Autodesk Inventor part; units mm, degrees
ref_plane "FDT_FRONT_XY" through (33, 0, 0) normal (1, 0, 0) x (0, 0, -1)
ref_plane "FDT_FRONT_YZ" through (33, 0, 0) normal (0, 0, -1) x (0, 1, 0)
ref_plane "FDT_FRONT_ZX" through (33, 0, 0) normal (0, 1, 0) x (1, 0, 0)
sketch "Sketch_22" plane through (0, 0, 0) normal (0, 0, 1) x (1, 0, 0)
  line L0 (33, 0) -> (0, 0)
  line L1 (0, 0) -> (0, 20.8)
  line L2 (0, 20.8) -> (0.6, 21.4)
  line L3 (0.6, 21.4) -> (3, 21.4)
  line L4 (3, 21.4) -> (3.6351, 22.5)
  line L5 (3.6351, 22.5) -> (27.3649, 22.5)
  line L6 (27.3649, 22.5) -> (27.8268, 21.7)
  arc A0 (27.8268, 21.7) -> (28.3464, 21.4) centre (28.3464, 22) ccw
  line L7 (28.3464, 21.4) -> (29.4, 21.4)
  arc A1 (29.4, 21.4) -> (30, 22) centre (29.4, 22) ccw
  line L8 (30, 22) -> (30, 22.5)
  line L9 (30, 22.5) -> (33, 22.5)
  line L10 (33, 22.5) -> (33, 0)
  line L11 (33, 0) -> (0, 0)
revolve "Revolution1" add sketch "Sketch_22" angle 360 about axis through (33, 0, 0) along (1, 0, 0)
thread "Thread1"
sketch "Sketch_2" plane through (33, 0, 0) normal (1, 0, 0) x (0, 0, -1)
  arc A0 (-12.7904, 32.5792) -> (12.7904, 32.5792) centre (0, 0) ccw
  arc A1 (12.6, 32.8585) -> (12.7904, 32.5792) centre (12.9, 32.8585) ccw
  line L0 (12.6, 32.8585) -> (12.6, 34.8)
  arc A2 (12.6, 34.8) -> (12.4, 35) centre (12.4, 34.8) ccw
  line L1 (12.4, 35) -> (-12.4, 35)
  arc A3 (-12.4, 35) -> (-12.6, 34.8) centre (-12.4, 34.8) ccw
  line L2 (-12.6, 34.8) -> (-12.6, 32.8585)
  arc A4 (-12.7904, 32.5792) -> (-12.6, 32.8585) centre (-12.9, 32.8585) ccw
extrude "Extrusion1" add sketch "Sketch_2" along normal blind 28
sketch "Sketch_3" plane through (0, 0, 0) normal (0, 0, 1) x (1, 0, 0)
  line L0 (599.2, 0) -> (61, 0)
  line L1 (61, 0) -> (61, 32.7)
  line L2 (61, 32.7) -> (599.2, 32.7)
  line L3 (599.2, 32.7) -> (599.2, 0)
  line L4 (599.2, 0) -> (61, 0)
revolve "Revolution2" add sketch "Sketch_3" angle 360 about axis through (599.2, 0, 0) along (1, 0, 0)
sketch "Sketch_16" plane through (599.2, 0, 0) normal (1, 0, 0) x (0, 0, -1)
  arc A0 (-12.7904, 32.5792) -> (12.7904, 32.5792) centre (0, 0) ccw
  arc A1 (12.6, 32.8585) -> (12.7904, 32.5792) centre (12.9, 32.8585) ccw
  line L0 (12.6, 32.8585) -> (12.6, 34.8)
  arc A2 (12.6, 34.8) -> (12.4, 35) centre (12.4, 34.8) ccw
  line L1 (12.4, 35) -> (-12.4, 35)
  arc A3 (-12.4, 35) -> (-12.6, 34.8) centre (-12.4, 34.8) ccw
  line L2 (-12.6, 34.8) -> (-12.6, 32.8585)
  arc A4 (-12.7904, 32.5792) -> (-12.6, 32.8585) centre (-12.9, 32.8585) ccw
extrude "Extrusion2" add sketch "Sketch_16" along normal blind 28
sketch "Sketch_5" plane through (0, 0, 0) normal (0, 0, 1) x (1, 0, 0)
  line L0 (660.2, 0) -> (627.2, 0)
  line L1 (627.2, 0) -> (627.2, 22.5)
  line L2 (627.2, 22.5) -> (630.2, 22.5)
  line L3 (630.2, 22.5) -> (630.2, 22)
  arc A0 (630.2, 22) -> (630.8, 21.4) centre (630.8, 22) ccw
  line L4 (630.8, 21.4) -> (631.8536, 21.4)
  arc A1 (631.8536, 21.4) -> (632.3732, 21.7) centre (631.8536, 22) ccw
  line L5 (632.3732, 21.7) -> (632.8351, 22.5)
  line L6 (632.8351, 22.5) -> (656.5649, 22.5)
  line L7 (656.5649, 22.5) -> (657.2, 21.4)
  line L8 (657.2, 21.4) -> (659.6, 21.4)
  line L9 (659.6, 21.4) -> (660.2, 20.8)
  line L10 (660.2, 20.8) -> (660.2, 0)
  line L11 (660.2, 0) -> (627.2, 0)
revolve "Revolution3" add sketch "Sketch_5" angle 360 about axis through (660.2, 0, 0) along (1, 0, 0)
thread "Thread2"
sketch "Sketch_6" plane through (0, 0, 0) normal (0, 1, 0) x (-1, 0, 0)
  line L0 (-628.2, -31.5) -> (-628.2, -10.5)
  line L1 (-628.2, -10.5) -> (-660.2, -10.5)
  line L2 (-660.2, -10.5) -> (-660.2, 10.5)
  line L3 (-660.2, 10.5) -> (-628.2, 10.5)
  line L4 (-628.2, 10.5) -> (-628.2, 31.5)
  line L5 (-628.2, 31.5) -> (-681.2, 31.5)
  line L6 (-681.2, 31.5) -> (-681.2, -31.5)
  line L7 (-681.2, -31.5) -> (-628.2, -31.5)
extrude "Extrusion3" cut sketch "Sketch_6" along normal mid plane 70
sketch "Sketch7" plane through (656.5649, -19.8997, -10.5) normal (0, 0, -1) x (-1, 0, 0)
  point P0 (12.3649, 19.8997)
hole "Hole1" at (644.2, 0, -10.5) direction (0, 0, 1) diameter 16 depth 21
sketch "Sketch8" plane through (33, 35, 12.4) normal (0, 1, 0) x (1, 0, 0)
  point P0 (13, 12.4)
hole "Hole2" at (46, 35, 0) direction (0, -1, 0) diameter 14.95 depth 17 countersink diameter 16.662 countersink angle 90
sketch "Sketch9" plane through (599.2, 35, 12.4) normal (0, 1, 0) x (1, 0, 0)
  point P0 (15, 12.4)
hole "Hole3" at (614.2, 35, 0) direction (0, -1, 0) diameter 14.95 depth 17 countersink diameter 16.662 countersink angle 90
sketch "Sketch_64" plane through (0, 0, 0) normal (0, 0, 1) x (1, 0, 0)
  line L0 (588.95, 0) -> (-12, 0)
  line L1 (-12, 0) -> (-12, 10)
  line L2 (-12, 10) -> (73.2, 10)
  line L3 (73.2, 10) -> (73.2, 31.5)
  line L4 (73.2, 31.5) -> (588.95, 31.5)
  line L5 (588.95, 31.5) -> (588.95, 0)
  line L6 (588.95, 0) -> (-12, 0)
revolve "Revolution4" cut sketch "Sketch_64" angle 360 about axis through (588.95, 0, 0) along (1, 0, 0)
ref_plane "FDT_FRONT_XY" through (33, 0, 0) normal (1, 0, 0) x (0, 0, -1)
ref_plane "FDT_FRONT_YZ" through (33, 0, 0) normal (0, 0, -1) x (0, 1, 0)
ref_plane "FDT_FRONT_ZX" through (33, 0, 0) normal (0, 1, 0) x (1, 0, 0)
ref_plane "FDT_QSFRONT_XY" through (46, 35, 0) normal (0, 1, 0) x (0, 0, 1)
ref_plane "FDT_QSFRONT_YZ" through (46, 35, 0) normal (0, 0, 1) x (1, 0, 0)
ref_plane "FDT_QSFRONT_ZX" through (46, 35, 0) normal (1, 0, 0) x (0, 1, 0)
ref_plane "FDT_QSREAR_XY" through (614.2, 35, 0) normal (0, 1, 0) x (0, 0, 1)
ref_plane "FDT_QSREAR_YZ" through (614.2, 35, 0) normal (0, 0, 1) x (1, 0, 0)
ref_plane "FDT_QSREAR_ZX" through (614.2, 35, 0) normal (1, 0, 0) x (0, 1, 0)
ref_plane "FDT_REAR_XY" through (627.2, 0, 0) normal (-1, 0, 0) x (0, 0, -1)
ref_plane "FDT_REAR_YZ" through (627.2, 0, 0) normal (0, 0, -1) x (0, -1, 0)
ref_plane "FDT_REAR_ZX" through (627.2, 0, 0) normal (0, -1, 0) x (-1, 0, 0)
ref_plane "FDT_SMBR1_XY" through (70.5, 0, 0) normal (-1, 0, 0) x (0, 0, 1)
ref_plane "FDT_SMBR1_YZ" through (70.5, 0, 0) normal (0, 0, 1) x (0, 1, 0)
ref_plane "FDT_SMBR1_ZX" through (70.5, 0, 0) normal (0, 1, 0) x (-1, 0, 0)
ref_plane "FDT_SMBR2_XY" through (589.7, 0, 0) normal (-1, 0, 0) x (0, 0, 1)
ref_plane "FDT_SMBR2_YZ" through (589.7, 0, 0) normal (0, 0, 1) x (0, 1, 0)
ref_plane "FDT_SMBR2_ZX" through (589.7, 0, 0) normal (0, 1, 0) x (-1, 0, 0)
ref_plane "FDT_SWIVELAXIS_XY" through (644.2, 0, 0) normal (0, 0, 1) x (1, 0, 0)
ref_plane "FDT_SWIVELAXIS_YZ" through (644.2, 0, 0) normal (1, 0, 0) x (0, 1, 0)
ref_plane "FDT_SWIVELAXIS_ZX" through (644.2, 0, 0) normal (0, 1, 0) x (0, 0, 1)
ref_plane "NUT_XY" through (8.5, 0, 0) normal (1, 0, 0) x (0, 0, -1)
ref_plane "NUT_YZ" through (8.5, 0, 0) normal (0, 0, -1) x (0, 1, 0)
ref_plane "NUT_ZX" through (8.5, 0, 0) normal (0, 1, 0) x (1, 0, 0)
ref_plane "ZR_XY" through (0, 0, 0) normal (-1, 0, 0) x (0, 0, -1)
ref_plane "ZR_YZ" through (0, 0, 0) normal (0, 0, -1) x (0, -1, 0)
ref_plane "ZR_ZX" through (0, 0, 0) normal (0, -1, 0) x (-1, 0, 0)
ref_plane "ZYL_XY" through (33, 0, 0) normal (1, 0, 0) x (0, 0, -1)
ref_plane "ZYL_YZ" through (33, 0, 0) normal (0, 0, -1) x (0, 1, 0)
ref_plane "ZYL_ZX" through (33, 0, 0) normal (0, 1, 0) x (1, 0, 0)
properties part number "193995 DSNU-63-500-P---(A----0-ZR)"
Check sheet for the modelled part. Datum: model origin and axes. Units: mm. A direction names the side the tool comes from. Give positions to 0.01 mm unless a question says otherwise; leave off trailing zeros. Order: outer loops, then holes, each group sorted by start corner. A loop starts at its lowest first (then second) coordinate and runs counter-clockwise, first axis right, second up. Notation, with made-up numbers: (49, -36.5) - (69, -36.5) arc R30 ccw to (69, -9.5) - close; hole circle Ø4 at (-35, 44). An arc over 180 degrees is marked (long way). Answer as CSV lines item,"result".
1. Section check C-C (x = 139.5). Record the boundary of the cut face in (y, z).
Result sheet:
outline,"circle Ø65.4 at (0, 0); hole circle Ø63 at (0, 0)"
2. Mould release check, pull along X, two halves, no side actions. Record for faces 1 (the face through (637, -5, 10.5)), 2 (the face through (38.59, 25.96, -0.97)), 3 (the face through (627.2, 0, -23)): released by +X, released by -X, zero draft, split by the parting line, or undercut.
Result sheet:
face 1,"zero draft"
face 2,"undercut"
face 3,"released by +X"
3. Scan lines: probe 1 along X at (y, z) = (24.5, 0.5); probe 2 along X at (y, z) = (-15.5, 25.5); probe 3 along X at (y, z) = (28, 5). Record each from-to range of solid material in increasing order. Write a range as from..to.
Result sheet:
probe 1,"33..38.54, 53.46..73.2, 588.95..606.74, 621.66..627.2"
probe 2,"33..73.2, 588.95..627.2"
probe 3,"33..40.44, 51.56..73.2, 588.95..608.64, 619.76..627.2"
4. Tool access check on faces 4 (the face through (621.5, 26, -1.6)), 5 (the face through (651, -5, -10.5)), 6 (the face through (1.8, -4.6, -20.9)), 7 (the face through (588.95, 0, 0)). Record the directions out of +Z, -Z, +X, -X, +Y, -Y that give a thin tool (end or side, any length) a straight path to the whole face; none if there is none.
Result sheet:
face 4,"+Y"
face 5,"-Z, +X, +Y, -Y"
face 6,"-X"
face 7,"none"
5. Go/stop test with flat-tipped pins: P1, Ø1, axis at x = 620, y = 33.5, coming from the -Z side; P2, Ø2, axis at x = 419, z = -9, coming from the -Y side; P3, Ø1, axis at y = -11.5, z = 18, coming from the +X side. Record where each tip stops, or that it passes through.
Result sheet:
P1,"z = -12.6"
P2,"y = -31.71"
P3,"x = 628.2"
6. Section check A-A (x = 644.2). Record the boundary of the cut face in (y, z).
Result sheet:
outline,"(-19.9, -10.5) - (-8, -10.5) - (-8, 10.5) - (-19.9, 10.5) arc R22.5 ccw to start; (8, -10.5) - (19.9, -10.5) arc R22.5 ccw to (19.9, 10.5) - (8, 10.5) - close"
